Verification items for the finished model (mm, model axes). Face numbers are marked on the shaded views. A direction names the side the tool comes from. Coordinates: 2 decimals unless noted, no trailing zeros. Write each loop counter-clockwise with the first axis right and the second up, starting at its lowest first coordinate (ties: lowest second). Pieces come first, ordered by that corner, then holes. Notation, with made-up numbers: M 26.5,37.5 L 65.5,37.5 A33 ccw 65.5,76.5 Z; hole C -24.75,9.5 d7. An arc over 180 degrees is marked long. Answer in a Markdown table with one row per item.
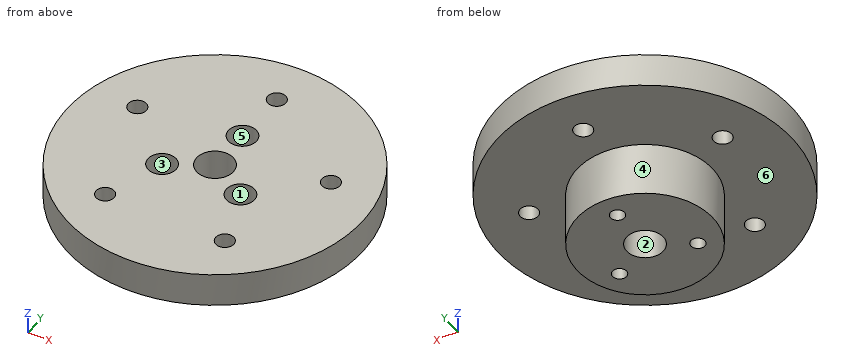
from build123d import *

# Parameters (mm, degrees)
F_4_0_4_HEAT_INSERT_M3_D         = 4
F_8_1_8_1_DURCHMESSER_BOHRUNG1_D = 8.1
SKIZZE8_R                        = 1.55
SCHNITT_LINEAR_AUSTRAGEN1_DEPTH  = 12
KREISMUSTER1_COUNT               = 5
SKIZZE9_R                        = 3.1
SCHNITT_LINEAR_AUSTRAGEN2_DEPTH  = 7.5


with BuildPart() as part:
    # Skizze1 → Rotation1 (revolve)
    with BuildSketch(Plane(origin=(0, 0, 0), x_dir=(0, 0, -1), z_dir=(1, 0, 0))):
        Polygon((0, 0), (19.5, 0), (19.5, 15), (7.5, 15), (7.5, 32.5), (0, 32.5), align=None)
    revolve(axis=Axis((0, 0, 0), (0, 0, 1)))

    # Ø4.0 (4) Heat Insert M3 (through all)
    with Locations(Plane.XY):
        with Locations((0, 22.5)):
            f_4_0_4_heat_insert_m3 = Hole(F_4_0_4_HEAT_INSERT_M3_D / 2)

    # Ø8.1 (8.1) Durchmesser Bohrung1 (through all)
    with Locations(Plane.XY):
        with Locations((0, 0)):
            Hole(F_8_1_8_1_DURCHMESSER_BOHRUNG1_D / 2)

    # Skizze8 → Schnitt-Linear austragen1 (cut)
    with BuildSketch(Plane(origin=(0, 0, -19.5), x_dir=(-1, 0, 0), z_dir=(0, 0, -1))):
        with Locations((0, 10)):
            Circle(SKIZZE8_R)
        with Locations((8.660254038, -5)):
            Circle(SKIZZE8_R)
        with Locations((-8.660254038, -5)):
            Circle(SKIZZE8_R)
    extrude(amount=-SCHNITT_LINEAR_AUSTRAGEN1_DEPTH, mode=Mode.SUBTRACT)

    # Kreismuster1: Ø4.0 (4) Heat Insert M3 ×5 about axis
    kreismuster1_axis = Axis((0, 0, 0), (0, 0, 1))
    for i in range(1, KREISMUSTER1_COUNT):
        add(f_4_0_4_heat_insert_m3.rotate(kreismuster1_axis, i * 360 / KREISMUSTER1_COUNT), mode=Mode.SUBTRACT)

    # Skizze9 → Schnitt-Linear austragen2 (cut)
    with BuildSketch(Plane.XY):
        with Locations((0, 10)):
            Circle(SKIZZE9_R)
        with Locations((8.660254038, -5)):
            Circle(SKIZZE9_R)
        with Locations((-8.660254038, -5)):
            Circle(SKIZZE9_R)
    extrude(amount=-SCHNITT_LINEAR_AUSTRAGEN2_DEPTH, mode=Mode.SUBTRACT)


solid = part.part
1) Sectioned sample at A-A (y = 0). Record the cut outline in (x, z), then the cut area to 3 significant figures.
Response values:
| item | result |
|---|---|
| outline | M -32.5,-7.5 L -15,-7.5 L -15,-19.5 L -4.05,-19.5 L -4.05,0 L -32.5,0 Z; M 4.05,-19.5 L 15,-19.5 L 15,-7.5 L 32.5,-7.5 L 32.5,0 L 4.05,0 Z |
| area | 690 mm² |
2) Release check for a two-part mould opening along Y. For the marked faces 3, 4, 5 and 6 record: +Y half, -Y half, draft (parallel to the pull), parting line (faces both ways), or undercut.
Response values:
| item | result |
|---|---|
| face 3 | undercut |
| face 4 | parting line |
| face 5 | undercut |
| face 6 | draft |
3) Thickness scan on L1, parallel to X at y = 8.5, z = -5.75; L2, parallel to Z at x = 25, y = 15; L3, parallel to Y at x = -11, z = -11.25. Record the ranges inside material, lowest first. Write a range as [from, to].
Response values:
| item | result |
|---|---|
| L1 | x = [-31.37, -22.67], [-20.13, -2.71], [2.71, 20.13], [22.67, 31.37] |
| L2 | z = [-7.5, 0] |
| L3 | y = [-10.2, 10.2] |
4) Sectioned sample at B-B (z = -4). Give the number of separate pieces and of enclosed holes in the cut face, then the cut area to 3 significant figures.
Response values:
| item | result |
|---|---|
| separate pieces | 1 |
| enclosed holes | 9 |
| area | 3,110 mm² |
5) Sectioned sample at C-C (z = -14.5). Record the cut outline in (x, y).
Response values:
| item | result |
|---|---|
| outline | C 0,0 d30; hole C -8.66,-5 d3.1; hole C 0,0 d8.1; hole C 0,10 d3.1; hole C 8.66,-5 d3.1 |
6) Depth check by flat-ended pin: pin 1 (5 mm diameter, centred on x = 8.66, y = -5, fed in from +Z); pin 2 (6 mm diameter, centred on y = 8, z = -6, fed in from -X); pin 3 (1 mm diameter, centred on y = 3.5, z = -12.5, fed in from -X). Enter the tip coordinate at first touch or a pass-through.
Response values:
| item | result |
|---|---|
| pin 1 | stops at z = -7.5 |
| pin 2 | stops at x = -32.11 |
| pin 3 | stops at x = -14.7 |
7) Tool access check on the marked faces 1 and 2. Record the directions out of +Z, -Z, +X, -X, +Y, -Y that give a thin tool (end or side, any length) a straight path to the whole face; none if there is none.
Response values:
| item | result |
|---|---|
| face 1 | +Z |
| face 2 | +Z, -Z |
8) Sectioned sample at D-D (y = 22.5). Record the cut outline in (x, z).
Response values:
| item | result |
|---|---|
| outline | M -23.45,-7.5 L -2,-7.5 L -2,0 L -23.45,0 Z; M 2,-7.5 L 23.45,-7.5 L 23.45,0 L 2,0 Z |
